Model file for the job. Use its own axes, mm. Face numbers are marked on the shaded views. A direction names the side the tool comes from. Round coordinates to 2 decimals unless told otherwise and drop trailing zeros. Loops run counter-clockwise (first coordinate to the right, second up) from the corner with the lowest first, then second, coordinate; pieces in that order, holes last. Notation, with made-up numbers: (27, 38.25) - (31, 38.25) arc R22 ccw to (31, 46.25) - close; hole circle Ø10 at (-38.5, 31.5). An arc over 180 degrees is marked (long way). Answer as a JSON object with one key per item and string values.
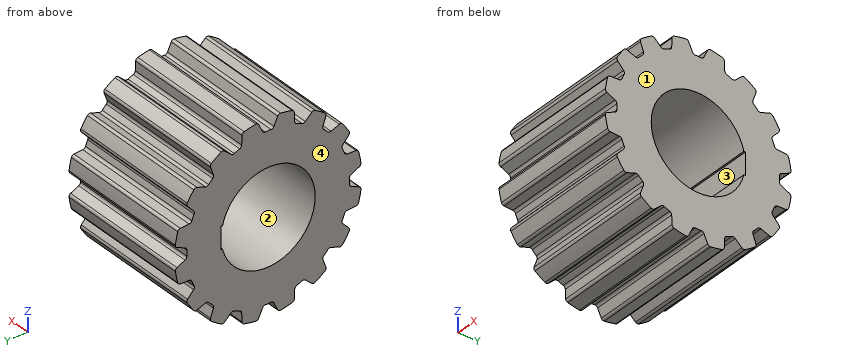
from build123d import *

# Parameters (mm, degrees)
CHAMFER_1_SIZE           = 1
SKETCH_4_W               = 3
SKETCH_4_H               = 1.630303969
CUT_EXTRUDE_1_DEPTH      = 43.109684421
CUT_EXTRUDE_2_REACH      = 44.11
PATTERN_CIRCULAR_3_COUNT = 16
SKETCH_7_R               = 23.358425388
CUT_EXTRUDE_3_DEPTH      = 20


with BuildPart() as part:
    # Sketch 1 → Revolve 1 (revolve)
    with BuildSketch(Plane.XY, mode=Mode.PRIVATE) as revolve_1_sk:
        Polygon((0, 5), (0, 12.681), (38.1, 12.681), (38.1, 6.3664), (6.65, 6.3664), (6.65, 5), align=None)
    revolve(revolve_1_sk.sketch.rotate(Axis((0, 0, 0), (1, 0, 0)), 90), axis=Axis((0, 0, 0), (1, 0, 0)))

    # Chamfer 1
    chamfer_1_edges = [part.edges().sort_by_distance(p)[0] for p in [
        (6.65, 0, -5),
        (0, 0, -5),
    ]]
    chamfer(chamfer_1_edges, length=CHAMFER_1_SIZE)

    # Sketch 4 → Cut-Extrude 1 (cut, through all)
    with BuildSketch(Plane.ZY):
        with Locations((0, 5.584847992)):
            Rectangle(SKETCH_4_W, SKETCH_4_H)
    extrude(amount=-CUT_EXTRUDE_1_DEPTH, mode=Mode.SUBTRACT)

    # Sketch 6 → Cut-Extrude 2 (cut, up to next)
    with BuildSketch(Plane(origin=(0, 0, 0), x_dir=(0, 0, -1), z_dir=(1, 0, 0)), mode=Mode.PRIVATE) as cut_extrude_2_sk1:
        with BuildLine():
            Line((1.285723043, 12.353105336), (0.776264221, 11.260567368))
            ThreePointArc((0.776264221, 11.260567368), (0.618819992, 11.084207877), (0.390175975, 11.02409741))
            ThreePointArc((0.390175975, 11.02409741), (0, 11.031), (-0.390175975, 11.02409741))
            ThreePointArc((-0.390175975, 11.02409741), (-0.618819992, 11.084207877), (-0.776264221, 11.260567368))
            Line((-0.776264221, 11.260567368), (-1.285723043, 12.353105336))
            ThreePointArc((-1.285723043, 12.353105336), (-1.447679281, 12.525850138), (-1.680477339, 12.569158958))
            ThreePointArc((-1.680477339, 12.569158958), (-1.868612982, 12.542569375), (-2.056329114, 12.513163931))
            Line((-2.056329114, 12.513163931), (-2.671802841, 13.8330516))
            ThreePointArc((-2.671802841, 13.8330516), (0, 14.088713461), (2.671802841, 13.8330516))
            Line((2.671802841, 13.8330516), (2.056329114, 12.513163931))
            ThreePointArc((2.056329114, 12.513163931), (1.868612982, 12.542569375), (1.680477339, 12.569158958))
            ThreePointArc((1.680477339, 12.569158958), (1.447679281, 12.525850138), (1.285723043, 12.353105336))
        make_face()
    cut_extrude_2_tool1 = extrude(cut_extrude_2_sk1.sketch, amount=CUT_EXTRUDE_2_REACH, mode=Mode.PRIVATE) & part.part
    cut_extrude_2 = cut_extrude_2_tool1.solids().sort_by_distance((0, 12.873618, 0))[0]
    add(cut_extrude_2, mode=Mode.SUBTRACT)

    # Pattern Circular 3: Cut-Extrude 2 ×16 about axis
    pattern_circular_3_axis = Axis((0, 0, 0), (1, 0, 0))
    for i in range(1, PATTERN_CIRCULAR_3_COUNT):
        add(cut_extrude_2.rotate(pattern_circular_3_axis, i * 360 / PATTERN_CIRCULAR_3_COUNT), mode=Mode.SUBTRACT)

    # Sketch 7 → Cut-Extrude 3 (cut)
    with BuildSketch(Plane.ZY):
        Circle(SKETCH_7_R)
    extrude(amount=-CUT_EXTRUDE_3_DEPTH, mode=Mode.SUBTRACT)


solid = part.part
1) Tool access for the marked faces 3 and 4: list every direction of +Z, -Z, +X, -X, +Y, -Y with a clear straight run to the whole face (end or side of a thin tool).
Values follow:
{"face 3": "+X, -X", "face 4": "+Z, -Z, -X, +Y, -Y"}
2) Two-plate mould, pull along Z, no slides. Class the marked faces 1 and 2: pulls with the +Z half, pulls with the -Z half, needs draft (parallel to the pull), parting line crosses it, or undercut.
Values follow:
{"face 1": "needs draft", "face 2": "undercut"}
3) Slice it at A-A on z = 0. List the corners of the cut face in (x, y).
Values follow:
{"outline": "(20, -11.03) - (38.1, -11.03) - (38.1, -6.37) - (20, -6.37) - close; (20, 6.4) - (38.1, 6.4) - (38.1, 11.03) - (20, 11.03) - close"}
4) Drop flat-ended pins along their axis: P1, Ø1, axis at x = 28, y = 7, coming from the -Z side; P2, Ø6, axis at x = 26.5, y = -9, coming from the -Z side; P3, Ø11.5, axis at y = 0, z = 0, coming from the +X side; P4, Ø4, axis at x = 29.5, y = -3.5, coming from the +Z side. Give the stop position or say it passes through.
Values follow:
{"P1": "z = -10.89", "P2": "z = -11.02", "P3": "through", "P4": "z = 12.57"}
5) Slice it at C-C on z = 7. List the corners of the cut face in (x, y).
Values follow:
{"outline": "(20, -10.57) - (38.1, -10.57) - (38.1, 10.57) - (20, 10.57) - close"}
6) Slice it at B-B on y = 0. List the corners of the cut face in (x, z), then the cut area to 3 significant figures.
Values follow:
{"outline": "(20, -11.03) - (38.1, -11.03) - (38.1, -6.37) - (20, -6.37) - close; (20, 6.37) - (38.1, 6.37) - (38.1, 11.03) - (20, 11.03) - close", "area": "169 mm²"}
7) Probe probe 1 along Z at (x, y) = (33, 0); probe 2 along Y at (x, z) = (30.25, 0); probe 3 along Z at (x, y) = (26.75, 1.5). List the from-to ranges inside material, lowest first.
Values follow:
{"probe 1": "-11.03 to -6.37, 6.37 to 11.03", "probe 2": "-11.03 to -6.37, 6.4 to 11.03", "probe 3": "-12.55 to -6.19, 6.19 to 12.55"}
